Autodesk Inventor part; units mm, degrees
ref_plane "YZ Plane" through (0, 0, 0) normal (1, 0, 0) x (0, 1, 0)
ref_plane "XZ Plane" through (0, 0, 0) normal (0, 1, 0) x (-1, 0, 0)
ref_plane "XY Plane" through (0, 0, 0) normal (0, 0, 1) x (1, 0, 0)
sketch "Sketch1" plane through (0, 0, 0) normal (0, 0, 1) x (1, 0, 0)
  circle A0 centre (0, 0) radius 41.148
  dimension "d0" = 82.296
extrude "Extrusion1" add sketch "Sketch1" against normal blind 152.4
sketch "Sketch2" plane through (0, 0, 0) normal (0, 0, 1) x (1, 0, 0)
  circle A0 centre (0, 0) radius 21.971
  dimension "d3" = 43.942
extrude "Extrusion2" cut sketch "Sketch2" against normal blind 152.4
sketch "Sketch3" plane through (0, 0, 0) normal (0, 0, 1) x (1, 0, 0)
  circle A0 centre (0, 0) radius 28.575
  dimension "d6" = 57.15
extrude "Extrusion3" cut sketch "Sketch3" against normal blind 24.892
sketch "Sketch4" plane through (0, 0, -152.4) normal (0, 0, -1) x (-1, 0, 0)
  circle A0 centre (0, 0) radius 28.575
  dimension "d9" = 57.15
extrude "Extrusion4" cut sketch "Sketch4" against normal blind 25.908
sketch "Sketch5" plane through (0, 0, 0) normal (0, 0, 1) x (1, 0, 0)
  circle A0 centre (0, 0) radius 41.148
  circle A1 centre (0, 0) radius 31.75
  dimension "d12" = 63.5
extrude "Extrusion5" cut sketch "Sketch5" against normal blind 177.8
sketch "Sketch6" plane through (0, 0, 0) normal (0, 0, 1) x (1, 0, 0)
  circle A0 centre (0, 0) radius 31.75
  circle A1 centre (0, 0) radius 41.148
  dimension "d15" = 82.296
extrude "Extrusion6" add sketch "Sketch6" against normal blind 6.35
sketch "Sketch7" plane through (0, 0, -152.4) normal (0, 0, -1) x (-1, 0, 0)
  circle A0 centre (0, 0) radius 31.75
  circle A1 centre (0, 0) radius 31.75
  circle A2 centre (0, 0) radius 41.148
extrude "Extrusion7" add sketch "Sketch7" against normal blind 6.35
sketch "Sketch8" plane through (0, 0, 0) normal (0, 0, 1) x (1, 0, 0)
  circle A0 centre (0, 36.449) radius 2.3813
  circle A1 centre (31.5658, 18.2245) radius 2.3813
  circle A2 centre (31.5658, -18.2245) radius 2.3813
  circle A3 centre (0, -36.449) radius 2.3813
  circle A4 centre (-31.5658, -18.2245) radius 2.3813
  circle A5 centre (-31.5658, 18.2245) radius 2.3813
  point P0 (0, 0)
  dimension "d20" = 4.7625
  dimension "d23" = 360
extrude "Extrusion8" cut sketch "Sketch8" against normal blind 177.8
properties part number "CombustionChamber4_4"
Input: part model. Units: mm. Frame: model coordinates. A direction names the side the tool comes from. Give positions to 0.01 mm unless a question says otherwise; leave off trailing zeros. Write each loop counter-clockwise with the first axis right and the second up, starting at its lowest first coordinate (ties: lowest second). Pieces come first, ordered by that corner, then holes.
Q1. Section C-C, the plane z = -48. Output: boundary loops of the cut face in (x, y), plus the area to 3 significant figures.
Q2. Pull-direction query (Z, two-part tool) for faces 4 (the face through (9, 28, 0)), 5 (the face through (9, 31, -146.05)), 6 (the face through (-33.945, -18.12, -149.181)); classes: pulls with the +Z half, pulls with the -Z half, needs draft (parallel to the pull), parting line crosses it, or undercut.
Q3. Section D-D, the plane x = 0. State how many separate pieces and enclosed holes the cut face has, plus the area to 3 significant figures.
Q4. Section A-A, the plane y = 0. Output: boundary loops of the cut face in (x, z) (3 decimals), plus the area to 3 significant figures.
Q5. Material intervals for probe 1 along Y at (x, z) = (0, -149.5) (3 decimals); probe 2 along Z at (x, y) = (4.5, -33.5); probe 3 along Y at (x, z) = (0, -142) (3 decimals), sorted ascending.
Q6. Section B-B, the plane x = -14. Output: boundary loops of the cut face in (y, z).
Q7. First-contact query: P1, Ø3, axis at x = 22, y = 16, coming from the +Z side; P2, Ø4, axis at y = 14.5, z = -134.5, coming from the -X side; P3, Ø3, axis at y = -21, z = -72.5, coming from the +X side; P4, Ø3, axis at x = 31.57, y = 18.22, coming from the +Z side. Flat tips, straight axial feed; report the tip coordinate or a pass-through.
Q8. Set-up query: faces 1 (the face through (33.766, -19.137, -149.181)), 2 (the face through (8, -21, -24.892)), 3 (the face through (-9, 31, -6.35)). Return all of +Z, -Z, +X, -X, +Y, -Y with unobstructed straight access to the full face (end or side cutting, diameter ignored); none if empty.
Filled in:
1. outline: circle Ø63.5 at (0, 0); hole circle Ø43.94 at (0, 0)
1. area: 1,650 mm2
2. face 4: pulls with the +Z half
2. face 5: undercut
2. face 6: needs draft
3. separate pieces: 6
3. enclosed holes: 0
3. area: 2,430 mm2
4. outline: (-41.148, -152.4) - (-28.575, -152.4) - (-28.575, -126.492) - (-21.971, -126.492) - (-21.971, -24.892) - (-28.575, -24.892) - (-28.575, 0) - (-41.148, 0) - (-41.148, -6.35) - (-31.75, -6.35) - (-31.75, -146.05) - (-41.148, -146.05) - close; (21.971, -126.492) - (28.575, -126.492) - (28.575, -152.4) - (41.148, -152.4) - (41.148, -146.05) - (31.75, -146.05) - (31.75, -6.35) - (41.148, -6.35) - (41.148, 0) - (28.575, 0) - (28.575, -24.892) - (21.971, -24.892) - close
4. area: 2,550 mm2
5. probe 1: y = -41.148 to -38.83, -34.068 to -28.575, 28.575 to 34.068, 38.83 to 41.148
5. probe 2: z = -152.4 to -146.05, -6.35 to 0
5. probe 3: y = -31.75 to -28.575, 28.575 to 31.75
6. outline: (-38.69, -152.4) - (-24.91, -152.4) - (-24.91, -126.49) - (-16.93, -126.49) - (-16.93, -24.89) - (-24.91, -24.89) - (-24.91, 0) - (-38.69, 0) - (-38.69, -6.35) - (-28.5, -6.35) - (-28.5, -146.05) - (-38.69, -146.05) - close; (16.93, -126.49) - (24.91, -126.49) - (24.91, -152.4) - (38.69, -152.4) - (38.69, -146.05) - (28.5, -146.05) - (28.5, -6.35) - (38.69, -6.35) - (38.69, 0) - (24.91, 0) - (24.91, -24.89) - (16.93, -24.89) - close
7. P1: stops at z = 0
7. P2: stops at x = -29.19
7. P3: stops at x = 25.06
7. P4: passes through
8. face 1: +Z, -Z
8. face 2: +Z
8. face 3: none
